Input: dimensioned drawing with shaded views. Units: mm. Origin: part minimum x, y, z. Round coordinates to 2 decimals unless told otherwise and drop trailing zeros. Loops run counter-clockwise (first coordinate to the right, second up) from the corner with the lowest first, then second, coordinate; pieces in that order, holes last. Notation, with made-up numbers: M 2.25,57.25 L 27.25,57.25 A26 cw 27.25,88.25 Z; hole C 58.25,56.5 d8. An arc over 180 degrees is marked long. Use one line per item in the form item = value. Start each with the question number.
Q1. Section query D-D, the plane x = 3. Output: boundary loops of the cut face in (y, z), and give its area (3 significant figures).
Q2. Section query C-C, the plane x = 19.5. Output: boundary loops of the cut face in (y, z), and give its area (3 significant figures).
Q3. Ray query, line 1 along Z through (x, y) = (29, 15); line 2 along Z through (x, y) = (24.5, 187); line 3 along X through (y, z) = (153, 13.75). Return the intervals inside material, ascending.
Q4. Section query A-A, the plane z = 12.7. Output: boundary loops of the cut face in (x, y).
Q5. First-contact query: P1, Ø8, axis at y = 121.826, z = 12.7, coming from the -X side; P2, Ø1.5, axis at x = 23.5, z = 15, coming from the -Y side. Flat tips, straight axial feed; report the tip coordinate or a pass-through.
Q6. Section query B-B, the plane y = 58.5. Output: boundary loops of the cut face in (x, z), and give its area (3 significant figures).
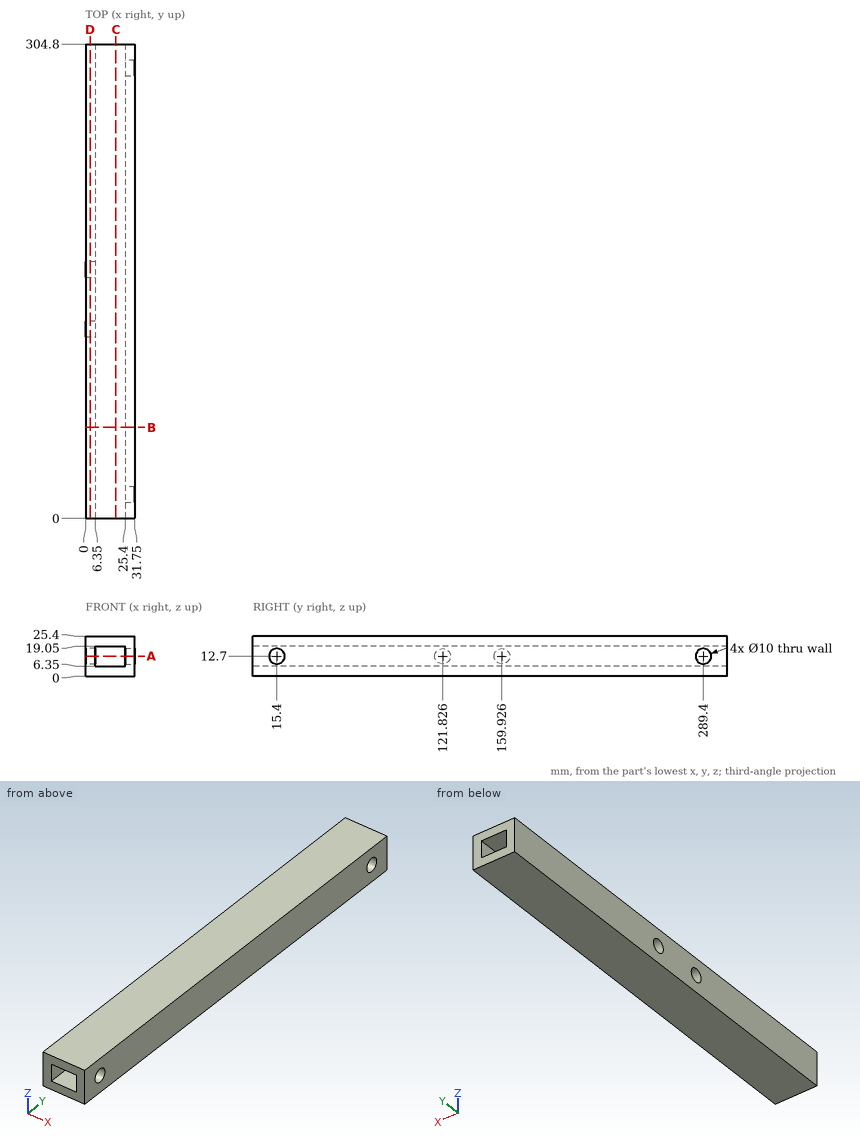
Results found:
q1.outline = M 0,0 L 304.8,0 L 304.8,25.4 L 0,25.4 Z; hole C 121.83,12.7 d10; hole C 159.93,12.7 d10
q1.area = 7,580 mm²
q2.outline = M 0,0 L 304.8,0 L 304.8,6.35 L 0,6.35 Z; M 0,19.05 L 304.8,19.05 L 304.8,25.4 L 0,25.4 Z
q2.area = 3,870 mm²
q3.line_1 = 0 to 7.72, 17.68 to 25.4
q3.line_2 = 0 to 6.35, 19.05 to 25.4
q3.line_3 = 0 to 6.35, 25.4 to 31.75
q4.outline = M 0,0 L 6.35,0 L 6.35,116.83 L 0,116.83 Z; M 0,126.83 L 6.35,126.83 L 6.35,154.93 L 0,154.93 Z; M 0,164.93 L 6.35,164.93 L 6.35,304.8 L 0,304.8 Z; M 25.4,0 L 31.75,0 L 31.75,10.4 L 25.4,10.4 Z; M 25.4,20.4 L 31.75,20.4 L 31.75,284.4 L 25.4,284.4 Z; M 25.4,294.4 L 31.75,294.4 L 31.75,304.8 L 25.4,304.8 Z
q5.P1 = 25.4
q5.P2 = through
q6.outline = M 0,0 L 31.75,0 L 31.75,25.4 L 0,25.4 Z; hole M 6.35,6.35 L 25.4,6.35 L 25.4,19.05 L 6.35,19.05 Z
q6.area = 565 mm²
